```python
from build123d import *

# Parameters (mm, degrees)
BOSS_EXTRUDE1_DEPTH = 88.3
SKETCH6_R           = 1.65
BOSS_EXTRUDE2_DEPTH = 8
CUT_EXTRUDE1_DEPTH  = 93.261259475
SKETCH8_W           = 61.3
SKETCH8_H           = 21.483950942
CUT_EXTRUDE2_DEPTH  = 93.118890571
SKETCH9_W           = 61.3
SKETCH9_H           = 11.699409457
CUT_EXTRUDE3_DEPTH  = 93.543511645
SKETCH10_R          = 1.65
CUT_EXTRUDE4_DEPTH  = 94.043055829
CHAMFER1_SIZE       = 8
CHAMFER1_SIZE2      = 3
CUT_EXTRUDE5_DEPTH  = 93.54351174
FILLET1_R           = 2
CUT_EXTRUDE6_DEPTH  = 3
CUT_EXTRUDE7_START  = -4.6
CUT_EXTRUDE7_DEPTH  = 4.6


with BuildPart() as part:
    # Sketch1 → Boss-Extrude1 (new body)
    with BuildSketch(Plane.ZY):
        with BuildLine():
            Line((-9.5, 8.25), (-9.5, -8.25))
            Line((-9.5, -8.25), (0, -8.25))
            ThreePointArc((0, -8.25), (8.25, 0), (0, 8.25))
            Line((0, 8.25), (-9.5, 8.25))
        make_face()
    extrude(amount=BOSS_EXTRUDE1_DEPTH)

    # Sketch6 → Boss-Extrude2 (add)
    with BuildSketch(Plane(origin=(0, 0, -9.5), x_dir=(-1, 0, 0), z_dir=(0, 0, -1))):
        with BuildLine():
            Line((17.15, -8.25), (17.15, 20))
            ThreePointArc((17.15, 20), (20.99096395, 24.863808737), (26.612654174, 22.254931867))
            Line((26.612654174, 22.254931867), (32.579554775, 10.446054507))
            ThreePointArc((32.579554775, 10.446054507), (34.053942202, 8.842964487), (36.149678114, 8.25))
            Line((36.149678114, 8.25), (52.150321886, 8.25))
            ThreePointArc((52.150321886, 8.25), (54.246057798, 8.842964487), (55.720445225, 10.446054507))
            Line((55.720445225, 10.446054507), (61.687345826, 22.254931867))
            ThreePointArc((61.687345826, 22.254931867), (67.30903605, 24.863808737), (71.15, 20))
            Line((71.15, 20), (71.15, -8.25))
            Line((71.15, -8.25), (17.15, -8.25))
        make_face()
        with Locations((22.15, 20)):
            Circle(SKETCH6_R, mode=Mode.SUBTRACT)
        with Locations(Location((66.15, 20, 0), (0, 0, 180))):
            Circle(SKETCH6_R, mode=Mode.SUBTRACT)
    extrude(amount=-BOSS_EXTRUDE2_DEPTH)

    # Sketch7 → Cut-Extrude1 (cut, through all)
    with BuildSketch(Plane.ZY.offset(88.3)):
        with BuildLine():
            Line((13.481907846, 13.481907846), (4.313351365, 4.313351365))
            ThreePointArc((4.313351365, 4.313351365), (-6.1, 0), (4.313351365, -4.313351365))
            Line((4.313351365, -4.313351365), (13.481907846, -13.481907846))
            Line((13.481907846, -13.481907846), (13.481907846, 13.481907846))
        make_face()
    extrude(amount=-CUT_EXTRUDE1_DEPTH, mode=Mode.SUBTRACT)

    # Sketch8 → Cut-Extrude2 (cut, through all)
    with BuildSketch(Plane.XY.offset(-1.5)):
        with Locations((-44.15, -2.491975471)):
            Rectangle(SKETCH8_W, SKETCH8_H)
    extrude(amount=CUT_EXTRUDE2_DEPTH, mode=Mode.SUBTRACT)

    # Sketch9 → Cut-Extrude3 (cut, through all)
    with BuildSketch(Plane(origin=(0, 0, -6.1), x_dir=(-1, 0, 0), z_dir=(0, 0, -1))):
        with Locations((44.15, -5.849704729)):
            Rectangle(SKETCH9_W, SKETCH9_H)
    extrude(amount=-CUT_EXTRUDE3_DEPTH, mode=Mode.SUBTRACT)

    # Sketch10 → Cut-Extrude4 (cut, through all)
    with BuildSketch(Plane(origin=(0, 0, -9.5), x_dir=(-1, 0, 0), z_dir=(0, 0, -1))):
        with Locations((22.15, 7)):
            Circle(SKETCH10_R)
        with Locations((66.15, 7)):
            Circle(SKETCH10_R)
    extrude(amount=-CUT_EXTRUDE4_DEPTH, mode=Mode.SUBTRACT)

    # Chamfer1
    chamfer1_edges = [part.edges().sort_by_distance(p)[0] for p in [
        (-44.15, -8.25, -6.1),
    ]]
    chamfer1_side = [part.faces().sort_by_distance(p)[0] for p in [
        (-44.15, -4.125, -6.1),
    ]]
    chamfer(chamfer1_edges, length=CHAMFER1_SIZE, length2=CHAMFER1_SIZE2, reference=chamfer1_side[0])

    # Sketch11 → Cut-Extrude5 (cut, through all)
    with BuildSketch(Plane(origin=(0, 0, -6.1), x_dir=(-1, 0, 0), z_dir=(0, 0, -1))):
        with BuildLine():
            Line((74.8, -8.25), (47.5958626, -1.828822614))
            ThreePointArc((47.5958626, -1.828822614), (44.15, -1.427659244), (40.7041374, -1.828822614))
            Line((40.7041374, -1.828822614), (13.5, -8.25))
            Line((13.5, -8.25), (13.5, -16.427659244))
            Line((13.5, -16.427659244), (74.8, -16.427659244))
            Line((74.8, -16.427659244), (74.8, -8.25))
        make_face()
    extrude(amount=CUT_EXTRUDE5_DEPTH, mode=Mode.SUBTRACT)

    # Fillet1
    fillet1_edges = [part.edges().sort_by_distance(p)[0] for p in [
        (-17.15, 8.25, -5.5),
        (-71.15, 8.25, -5.5),
    ]]
    fillet(fillet1_edges, radius=FILLET1_R)

    # Sketch12 → Cut-Extrude6 (cut)
    with BuildSketch(Plane(origin=(0, 0, -9.5), x_dir=(-1, 0, 0), z_dir=(0, 0, -1))):
        Polygon((22.15, 16.651368439), (25.05, 18.325684219), (25.05, 21.674315781), (22.15, 23.348631561), (19.25, 21.674315781), (19.25, 18.325684219), align=None)
        Polygon((66.15, 16.651368439), (69.05, 18.325684219), (69.05, 21.674315781), (66.15, 23.348631561), (63.25, 21.674315781), (63.25, 18.325684219), align=None)
    extrude(amount=-CUT_EXTRUDE6_DEPTH, mode=Mode.SUBTRACT)

    # Sketch13 → Cut-Extrude7 (cut)
    with BuildSketch(Plane.XY.offset(-1.5).offset(CUT_EXTRUDE7_START)):
        with BuildLine():
            Line((-69.3, 7), (-69.3, -2.12397244))
            Line((-69.3, -2.12397244), (-63, -2.12397244))
            Line((-63, -2.12397244), (-63, 7))
            ThreePointArc((-63, 7), (-66.15, 10.15), (-69.3, 7))
        make_face()
        with BuildLine():
            Line((-25.3, 7), (-25.3, -2.12397244))
            Line((-25.3, -2.12397244), (-19, -2.12397244))
            Line((-19, -2.12397244), (-19, 7))
            ThreePointArc((-19, 7), (-22.15, 10.15), (-25.3, 7))
        make_face()
    extrude(amount=CUT_EXTRUDE7_DEPTH, mode=Mode.SUBTRACT)


solid = part.part
```
The model under review builds one solid part; all positions refer to its coordinate system, in mm. A direction names the side the tool comes from. Coordinates: 2 decimals unless noted, no trailing zeros. Write each loop counter-clockwise with the first axis right and the second up, starting at its lowest first coordinate (ties: lowest second). Pieces come first, ordered by that corner, then holes. Notation, with made-up numbers: (52.5, -16) - (68.5, -16) arc R16 ccw to (68.5, 14) - close; hole circle Ø9 at (-17, 8). An arc over 180 degrees is marked (long way). Answer in a Markdown table with one row per item. Add a question column.
Q1. Consider section B-B on y = 14. Give the boundary of the cut face in (x, z), then the cut area to 3 significant figures.
Q2. Consider section A-A on z = 1.75. Give the boundary of the cut face in (x, y), then the cut area to 3 significant figures.
Q3. Consider section C-C on x = -76.5. Give the boundary of the cut face in (y, z), then the cut area to 3 significant figures.
Q4. For faces 1 (the face through (-20.68, 17.5, -8.02)), 2 (the face through (-13.5, -6, -3)), 3 (the face through (-58.37, -4.37, -8.39)), list the 3-axis set-ups (+Z, -Z, +X, -X, +Y, -Y) from which the entire face can be reached by the end or side of a thin tool; tool diameter is ignored.
Q5. Consider section D-D on y = 3.5. Give the boundary of the cut face in (x, z).
Q6. Clearance check with flat-ended pins moving along their axes: pin 1 (3 mm diameter, centred on x = -66.15, y = 20, fed in from -Z); pin 2 (3.5 mm diameter, centred on y = 4.5, z = -3.5, fed in from -X); pin 3 (2.5 mm diameter, centred on y = 20, z = -8.5, fed in from +X); pin 4 (6.5 mm diameter, centred on x = -40, z = -5.5, fed in from +Y). State where each tip first meets the part, or that it passes through.
Q7. To check wall thickness, follow line 1 along Y through (x, z) = (-66.15, -3.7); line 2 along Y through (x, z) = (-66.15, -8.7); line 3 along X through (y, z) = (19, -5.75). State the ranges of each line that lie inside material, in increasing order. Write a range as from..to.
Q8. Draft analysis for pull direction X (two halves, no side actions). For faces 4 (the face through (0, 0, -7)), 5 (the face through (-64.576, 19.504, -4.035)), 6 (the face through (-82, -8.25, -5)), state which applies: +X half, -X half, draft (parallel to the pull), parting line (faces both ways), or undercut.
Answers below:
| question | item | result |
|---|---|---|
| 1 | outline | (-71.15, -9.5) - (-57.52, -9.5) - (-57.52, -1.5) - (-71.15, -1.5) - close; (-30.78, -9.5) - (-17.15, -9.5) - (-17.15, -1.5) - (-30.78, -1.5) - close |
| 1 | area | 218 mm² |
| 2 | outline | (-88.3, -8.06) - (-74.8, -8.06) - (-74.8, -5.84) - (-88.3, -5.84) - close; (-88.3, 5.84) - (-74.8, 5.84) - (-74.8, 8.06) - (-88.3, 8.06) - close; (-13.5, -8.06) - (0, -8.06) - (0, -5.84) - (-13.5, -5.84) - close; (-13.5, 5.84) - (0, 5.84) - (0, 8.06) - (-13.5, 8.06) - close |
| 2 | area | 120 mm² |
| 3 | outline | (-8.25, -9.5) - (8.25, -9.5) - (8.25, 0) arc R8.25 ccw to (5.83, 5.83) - (4.31, 4.31) arc R6.1 cw (long way) to (-4.31, 4.31) - (-5.83, 5.83) arc R8.25 ccw to (-8.25, 0) - close |
| 3 | area | 123 mm² |
| 4 | face 1 | -Z |
| 4 | face 2 | +Z, -Y |
| 4 | face 3 | +Z, -Z, -Y |
| 5 | outline | (-88.3, -9.5) - (0, -9.5) - (0, -5) - (-19, -5) - (-19, -6.1) - (-25.3, -6.1) - (-25.3, -5) - (-63, -5) - (-63, -6.1) - (-69.3, -6.1) - (-69.3, -5) - (-88.3, -5) - close |
| 6 | pin 1 | through |
| 6 | pin 2 | x = -88.3 |
| 6 | pin 3 | x = -17.15 |
| 6 | pin 4 | y = 8.25 |
| 7 | line 1 | 10.15..18.35, 21.65..25 |
| 7 | line 2 | -6.21..5.35, 8.65..16.65, 23.35..25 |
| 7 | line 3 | -71.15..-67.46, -64.84..-60.04, -28.26..-23.46, -20.84..-17.15 |
| 8 | face 4 | +X half |
| 8 | face 5 | undercut |
| 8 | face 6 | draft |
